```python
from build123d import *

# Parameters (mm, degrees)
EXTRUDE_THIN1_DEPTH                   = 137.50025
EXTRUDE_THIN1_DEPTH_BACK              = 213.5
BOSS_EXTRUDE1_DEPTH                   = 212.50025
BOSS_EXTRUDE1_DEPTH_BACK              = 288.5
SKETCH3_OUTSIDE_W                     = 604.182
SKETCH3_OUTSIDE_H                     = 156.652
SKETCH3_OUTSIDE_W_2                   = 500
SKETCH3_OUTSIDE_H_2                   = 100
CUT_EXTRUDE1_DEPTH                    = 47.972186303
F_1_4_20_TAPPED_HOLE1_D               = 5.1054
F_1_4_20_TAPPED_HOLE1_DEPTH           = 16.51
F_1_4_20_TAPPED_HOLE1_TIP             = 1.533816902
F_1_4_20_TAPPED_HOLE1_ON_FACE_2_D     = 5.1054
F_1_4_20_TAPPED_HOLE1_ON_FACE_2_DEPTH = 16.51
F_1_4_20_TAPPED_HOLE1_ON_FACE_2_TIP   = 1.533816902
SKETCH5_OUTSIDE_W                     = 148.686
SKETCH5_OUTSIDE_H                     = 156.454
CUT_EXTRUDE2_DEPTH                    = 13
FILLET3_R                             = 2.1
FILLET4_R                             = 2.1
CHAMFER1_SIZE                         = 0.5


with BuildPart() as part:
    # Sketch1 → Extrude-Thin1 (new body, two sides)
    with BuildSketch(Plane.XY) as extrude_thin1_sk:
        with BuildLine():
            Line((-1, 29.097280522), (-1, 77.801426037))
            ThreePointArc((-1, 77.801426037), (-1.350622843, 78.7652373), (-2.238576202, 79.27846957))
            Line((-2.238576202, 79.27846957), (-14.558703222, 81.459024393))
            ThreePointArc((-14.558703222, 81.459024393), (-15.894736772, 81.028505528), (-16.289731153, 79.68154169))
            Line((-16.289731153, 79.68154169), (-16.133756175, 78.918587006))
            ThreePointArc((-16.133756175, 78.918587006), (-16.425245764, 77.689683446), (-17.55197675, 77.119028185))
            Line((-17.55197675, 77.119028185), (-31.176844121, 76.652024665))
            ThreePointArc((-31.176844121, 76.652024665), (-32.394172227, 75.953136676), (-32.500485503, 74.55348328))
            Line((-32.500485503, 74.55348328), (-32.189291755, 73.839630008))
            ThreePointArc((-32.189291755, 73.839630008), (-32.21890818, 72.576976846), (-33.20237149, 71.784531227))
            Line((-33.20237149, 71.784531227), (-46.048094305, 68.590520727))
            ThreePointArc((-46.048094305, 68.590520727), (-47.095522717, 67.648327863), (-46.899674591, 66.2531658))
            Line((-46.899674591, 66.2531658), (-20.221033316, 29.533166286))
            ThreePointArc((-20.221033316, 29.533166286), (-19.7411642, 29.106506164), (-19.126852316, 28.919599404))
            Line((-19.126852316, 28.919599404), (-2.619344492, 27.602035762))
            ThreePointArc((-2.619344492, 27.602035762), (-1.482408908, 27.995233168), (-1, 29.097280522))
        make_face()
        with BuildLine():
            Line((-1.27, 29.097280522), (-1.27, 77.801426037))
            ThreePointArc((-1.27, 77.801426037), (-1.557510731, 78.591751273), (-2.285632486, 79.012601734))
            Line((-2.285632486, 79.012601734), (-14.605759506, 81.193156557))
            ThreePointArc((-14.605759506, 81.193156557), (-15.701307017, 80.840131088), (-16.025202409, 79.735620741))
            Line((-16.025202409, 79.735620741), (-15.869227431, 78.972666057))
            ThreePointArc((-15.869227431, 78.972666057), (-16.213185147, 77.522559856), (-17.542727709, 76.849186648))
            Line((-17.542727709, 76.849186648), (-31.16759508, 76.382183127))
            ThreePointArc((-31.16759508, 76.382183127), (-32.165804128, 75.809094976), (-32.252981014, 74.661379192))
            Line((-32.252981014, 74.661379192), (-31.941787266, 73.94752592))
            ThreePointArc((-31.941787266, 73.94752592), (-31.976734648, 72.457595189), (-33.137221353, 71.522509358))
            Line((-33.137221353, 71.522509358), (-45.982944168, 68.328498858))
            ThreePointArc((-45.982944168, 68.328498858), (-46.841835466, 67.55590071), (-46.681240003, 66.411867819))
            Line((-46.681240003, 66.411867819), (-20.002598727, 29.691868304))
            ThreePointArc((-20.002598727, 29.691868304), (-19.609106053, 29.342007004), (-19.105370308, 29.188743461))
            Line((-19.105370308, 29.188743461), (-2.597862483, 27.871179818))
            ThreePointArc((-2.597862483, 27.871179818), (-1.665575304, 28.193601692), (-1.27, 29.097280522))
        make_face(mode=Mode.SUBTRACT)
    extrude(amount=EXTRUDE_THIN1_DEPTH)
    extrude(extrude_thin1_sk.sketch, amount=-EXTRUDE_THIN1_DEPTH_BACK)


with BuildPart() as body_2:
    # Sketch2 → Boss-Extrude1 (new body, two sides)
    with BuildSketch(Plane.XY) as boss_extrude1_sk:
        with BuildLine():
            Line((-46.68124, 66.411867814), (-20.002598727, 29.691868304))
            ThreePointArc((-20.002598727, 29.691868304), (-19.609106053, 29.342007004), (-19.105370308, 29.188743461))
            Line((-19.105370308, 29.188743461), (-2.597862483, 27.871179818))
            ThreePointArc((-2.597862483, 27.871179818), (-1.665575304, 28.193601692), (-1.27, 29.097280522))
            Line((-1.27, 29.097280522), (-1.27, 77.801426032))
            Line((-1.27, 77.801426032), (-1.27, 77.950492716))
            ThreePointArc((-1.27, 77.950492716), (-1.551343626, 78.723865476), (-2.263847169, 79.135688695))
            Line((-2.263847169, 79.135688695), (-14.583974189, 81.316243518))
            ThreePointArc((-14.583974189, 81.316243518), (-15.79085783, 80.927341477), (-16.14766942, 79.710584143))
            Line((-16.14766942, 79.710584143), (-15.991694442, 78.947629459))
            ThreePointArc((-15.991694442, 78.947629459), (-16.311361359, 77.599931889), (-17.547009673, 76.974113285))
            Line((-17.547009673, 76.974113285), (-31.171877043, 76.507109765))
            ThreePointArc((-31.171877043, 76.507109765), (-32.271530099, 75.875780948), (-32.367566426, 74.611427381))
            Line((-32.367566426, 74.611427381), (-32.056372677, 73.897574109))
            ThreePointArc((-32.056372677, 73.897574109), (-32.088852024, 72.512864474), (-33.167383454, 71.643815779))
            Line((-33.167383454, 71.643815779), (-46.013106268, 68.449805279))
            ThreePointArc((-46.013106268, 68.449805279), (-46.895812164, 67.655785195), (-46.730763849, 66.480031545))
            Line((-46.730763849, 66.480031545), (-46.68124, 66.411867814))
        make_face()
    extrude(amount=BOSS_EXTRUDE1_DEPTH)
    extrude(boss_extrude1_sk.sketch, amount=-BOSS_EXTRUDE1_DEPTH_BACK)

    # Sketch3 outside → Cut-Extrude1 (cut, through all)
    with BuildSketch(Plane(origin=(0, 0, 0), x_dir=(0, 0, -1), z_dir=(1, 0, 0))):
        with Locations((38, 54.602)):
            Rectangle(SKETCH3_OUTSIDE_W, SKETCH3_OUTSIDE_H)
        with Locations((37.999875, 53.523886616)):
            Rectangle(SKETCH3_OUTSIDE_W_2, SKETCH3_OUTSIDE_H_2, mode=Mode.SUBTRACT)
    extrude(amount=-CUT_EXTRUDE1_DEPTH, mode=Mode.SUBTRACT)

    # 1/4-20 Tapped Hole1
    with Locations(Plane(origin=(-13.27, 66.023886616, 212.000125), x_dir=(1, 0, 0), z_dir=(0, 0, 1))):
        with Locations((0, 0), (0, -25)):
            Hole(F_1_4_20_TAPPED_HOLE1_D / 2, depth=F_1_4_20_TAPPED_HOLE1_DEPTH)
            with Locations((0, 0, -(F_1_4_20_TAPPED_HOLE1_DEPTH + F_1_4_20_TAPPED_HOLE1_TIP / 2))):  # 118° drill point
                Cone(0, F_1_4_20_TAPPED_HOLE1_D / 2, F_1_4_20_TAPPED_HOLE1_TIP, mode=Mode.SUBTRACT)

    # 1/4-20 Tapped Hole1 on face 2
    with Locations(Plane(origin=(-13.27, 66.023886616, -287.999875), x_dir=(-1, 0, 0), z_dir=(0, 0, -1))):
        with Locations((0, 0), (0, -25)):
            Hole(F_1_4_20_TAPPED_HOLE1_ON_FACE_2_D / 2, depth=F_1_4_20_TAPPED_HOLE1_ON_FACE_2_DEPTH)
            with Locations((0, 0, -(F_1_4_20_TAPPED_HOLE1_ON_FACE_2_DEPTH + F_1_4_20_TAPPED_HOLE1_ON_FACE_2_TIP / 2))):  # 118° drill point
                Cone(0, F_1_4_20_TAPPED_HOLE1_ON_FACE_2_D / 2, F_1_4_20_TAPPED_HOLE1_ON_FACE_2_TIP, mode=Mode.SUBTRACT)

    # Sketch5 outside → Cut-Extrude2 (cut)
    with BuildSketch(Plane(origin=(0, 0, -287.999875), x_dir=(-1, 0, 0), z_dir=(0, 0, -1))):
        with Locations((24.121, 54.602)):
            Rectangle(SKETCH5_OUTSIDE_W, SKETCH5_OUTSIDE_H)
        with BuildLine():
            Line((2.57, 29.17309026), (18.969817109, 30.482058458))
            Line((18.969817109, 30.482058458), (45.647739584, 67.201068629))
            Line((45.647739584, 67.201068629), (32.853697609, 70.382229004))
            ThreePointArc((32.853697609, 70.382229004), (30.922831311, 71.938063902), (30.864684396, 74.417072944))
            Line((30.864684396, 74.417072944), (31.208213492, 75.205100887))
            Line((31.208213492, 75.205100887), (17.502477256, 75.674876254))
            ThreePointArc((17.502477256, 75.674876254), (15.290328755, 76.79526275), (14.718037528, 79.208010073))
            Line((14.718037528, 79.208010073), (14.890219467, 80.05024143))
            Line((14.890219467, 80.05024143), (2.57, 77.869670245))
            Line((2.57, 77.869670245), (2.57, 29.17309026))
        make_face(mode=Mode.SUBTRACT)
    extrude(amount=-CUT_EXTRUDE2_DEPTH, mode=Mode.SUBTRACT)

    # Fillet3
    fillet3_edges = [body_2.edges().sort_by_distance(p)[0] for p in [
        (-31.208213492, 75.205100887, -281.499875),
    ]]
    fillet(fillet3_edges, radius=FILLET3_R)

    # Fillet4
    fillet4_edges = [body_2.edges().sort_by_distance(p)[0] for p in [
        (-2.57, 29.17309026, -281.499875),
        (-18.969817109, 30.482058458, -281.499875),
        (-2.57, 77.869670245, -281.499875),
        (-45.647739584, 67.201068629, -281.499875),
        (-14.890219467, 80.05024143, -281.499875),
    ]]
    fillet(fillet4_edges, radius=FILLET4_R)

    # Chamfer1
    chamfer1_edges = [body_2.edges().sort_by_distance(p)[0] for p in [
        (-15.720977232, 76.353272794, -287.999875),
        (-31.252174207, 71.416195634, -287.999875),
        (-23.046962204, 75.484834478, -287.999875),
        (-30.023249286, 74.661893082, -287.999875),
        (-2.57, 53.778047874, -287.999875),
        (-8.307997228, 78.885245613, -287.999875),
        (-11.421630112, 29.879592183, -287.999875),
        (-31.677250598, 47.972340168, -287.999875),
        (-37.738977535, 69.167533996, -287.999875),
        (-13.844088825, 79.272536107, -287.999875),
        (-44.090657237, 66.633768979, -287.999875),
        (-3.06087198, 77.458049098, -287.999875),
        (-18.866214572, 30.666814075, -287.999875),
        (-3.245372471, 29.904516124, -287.999875),
    ]]
    chamfer(chamfer1_edges, length=CHAMFER1_SIZE)


solid = body_2.part
```
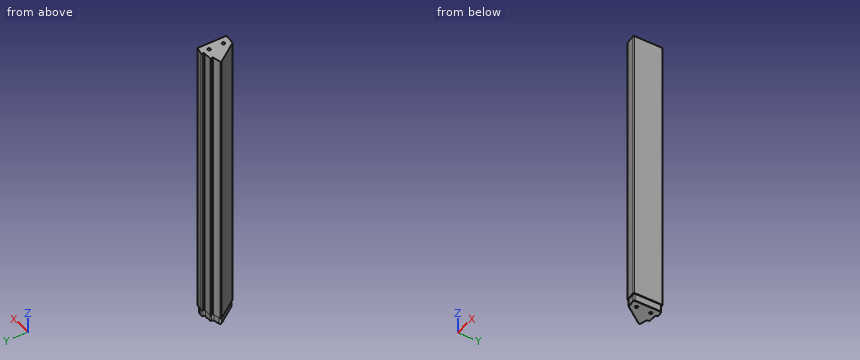
Verification items for the finished model (mm, model axes). Give positions to 0.01 mm unless a question says otherwise; leave off trailing zeros. Order: outer loops, then holes, each group sorted by start corner. A loop starts at its lowest first (then second) coordinate and runs counter-clockwise, first axis right, second up. Notation, with made-up numbers: (-23, -14) - (-11, -14) arc R15 cw to (-11, 11) - close; hole circle Ø9 at (5.25, 33). An arc over 180 degrees is marked (long way). Answer as CSV lines item,"result". Start each with the question number.
Item 1: Section check A-A, the plane z = -132.5. Record the boundary of the cut face in (x, y) (1 decimal), plus the area to 3 significant figures.
Item 2: Gauge pin test, flat ends, axial feed: pin 1 (4.5 mm diameter, centred on x = -13.27, y = 66.02, fed in from -Z); pin 2 (6 mm diameter, centred on y = 55, z = -70.5, fed in from -X); pin 3 (3 mm diameter, centred on x = -11.5, z = -25.5, fed in from +Y). Record the tip position at first contact, or that the pin passes through.
Item 3: Material ranges on L1, parallel to Y at x = -13, z = 203; L2, parallel to Y at x = -13, z = -276; L3, parallel to X at y = 45, z = 64, recorded low to high.
Filled in:
1,outline,"(-46.7, 66.5) - (-20, 29.7) arc R1.2 ccw to (-19.1, 29.2) - (-2.6, 27.9) arc R1.2 ccw to (-1.3, 29.1) - (-1.3, 78) arc R1.2 ccw to (-2.3, 79.1) - (-14.6, 81.3) arc R1.4 ccw to (-16.1, 79.7) - (-16, 78.9) arc R1.6 cw to (-17.5, 77) - (-31.2, 76.5) arc R1.4 ccw to (-32.4, 74.6) - (-32.1, 73.9) arc R1.6 cw to (-33.2, 71.6) - (-46, 68.4) arc R1.3 ccw to start"
1,area,"1,620 mm^2"
2,pin 1,"z = -271.31"
2,pin 2,"x = -40.57"
2,pin 3,"y = 81.04"
3,L1,"28.7 to 38.49, 43.56 to 63.49, 68.56 to 81.04"
3,L2,"30.01 to 38.49, 43.56 to 63.49, 68.56 to 79.6"
3,L3,"-31.12 to -1.27"
